Autodesk Fusion 360 part; units mm, degrees
sketch "Sketch1" plane through (0, 0, 0) normal (0, 0, 1) x (1, 0, 0)
  circle A0 centre (0, 0) radius 12.45
  dimension "d1" = 24.9
extrude "Extrude1" add sketch "Sketch1" along normal blind 18
sketch "Sketch2" plane through (0, 0, 18) normal (0, 0, 1) x (-1, 0, 0)
  circle A0 centre (0, 0) radius 12.45
  line L0 (0, 0) -> (0, -12.45)
  line L1 (0, 0) -> (-12.45, 0)
  line L2 (0, 0) -> (0, 12.45)
  line L3 (0, 0) -> (12.45, 0)
  line L4 (-12.45, 0) -> (-2.45, 0)
  circle A1 centre (-7.45, 0) radius 5
  line L5 (12.45, 0) -> (2.45, 0)
  line L6 (0, 12.45) -> (0, 2.45)
  line L7 (0, -12.45) -> (0, -2.45)
  circle A2 centre (0, -7.45) radius 5
  circle A3 centre (7.45, 0) radius 5
  circle A4 centre (0, 7.45) radius 5
  circle A5 centre (-7.45, 0) radius 3.75
  circle A6 centre (0, -7.45) radius 3.75
  circle A7 centre (0, 7.45) radius 3.75
  circle A8 centre (7.45, 0) radius 3.75
  circle A9 centre (-7.45, 0) radius 1
  circle A10 centre (0, -7.45) radius 1
  circle A11 centre (0, 7.45) radius 1
  circle A12 centre (7.45, 0) radius 1
  line L8 (-12.45, 0) -> (-12.45, -2.5)
  line L9 (-12.45, 0) -> (-12.45, 2.5)
  line L10 (-12.45, 2.5) -> (-11.7801, 2.5)
  line L11 (-12.45, -2.5) -> (-11.7801, -2.5)
  line L12 (0, -12.45) -> (-2.5, -12.45)
  line L13 (0, -12.45) -> (2.5, -12.45)
  line L14 (-2.5, -12.45) -> (-2.5, -11.7801)
  line L15 (12.45, 0) -> (12.45, -2.5)
  line L16 (12.45, 0) -> (12.45, 2.5)
  line L17 (12.45, 2.5) -> (10.2451, 2.5)
  line L18 (12.45, -2.5) -> (10.2451, -2.5)
  line L19 (2.5, -12.45) -> (2.5, -11.7801)
  line L20 (-2.5, -12.45) -> (-3.75, -12.45)
  line L21 (-3.75, -12.45) -> (-3.75, -10.7572)
  line L22 (2.5, -12.45) -> (3.75, -12.45)
  line L23 (3.75, -12.45) -> (3.75, -10.7572)
  line L24 (-3.75, -10.7572) -> (-3.75, -7.45)
  line L25 (2.5, -11.7801) -> (2.5, -10.2451)
  line L26 (-2.5, -11.7801) -> (-2.5, -10.2451)
  line L27 (3.75, -10.7572) -> (3.75, -7.45)
  line L28 (12.45, -2.5) -> (12.45, -3.75)
  line L29 (12.45, -3.75) -> (7.45, -3.75)
  line L30 (12.45, 1.25) -> (12.45, 2.5)
  line L31 (12.45, 2.5) -> (10.2451, 2.5)
  line L32 (12.45, 2.5) -> (12.45, 3.75)
  line L33 (12.45, 3.75) -> (7.45, 3.75)
  line L34 (0, 12.45) -> (-2.5, 12.45)
  line L35 (0, 12.45) -> (2.5, 12.45)
  line L36 (2.5, 12.45) -> (2.5, 10.2451)
  line L37 (2.5, 12.45) -> (3.75, 12.45)
  line L38 (3.75, 12.45) -> (3.75, 7.45)
  line L39 (-3.75, 7.45) -> (-3.75, 12.45)
  line L40 (-3.75, 12.45) -> (-2.5, 12.45)
  line L41 (-2.5, 12.45) -> (-2.5, 10.2451)
  line L42 (-11.7801, 2.5) -> (-10.2451, 2.5)
  line L43 (-11.7801, -2.5) -> (-10.2451, -2.5)
  line L44 (-12.45, -2.5) -> (-12.45, -3.75)
  line L45 (-12.45, 2.5) -> (-12.45, 3.75)
  line L46 (-12.45, 3.75) -> (-7.45, 3.75)
  line L47 (-12.45, -3.75) -> (-7.45, -3.75)
  dimension "d4" = 10
  dimension "d5" = 10
  dimension "d6" = 10
  dimension "d7" = 10
  dimension "d8" = 7.5
  dimension "d9" = 7.5
  dimension "d10" = 7.5
  dimension "d11" = 7.5
  dimension "d12" = 2
  dimension "d13" = 2
  dimension "d14" = 2
  dimension "d15" = 2
  dimension "d16" = 2.5
  dimension "d17" = 2.5
  dimension "d18" = 2.5
  dimension "d19" = 2.5
  dimension "d20" = 2.5
  dimension "d21" = 2.5
  dimension "d22" = 1.25
  dimension "d23" = 1.25
  dimension "d24" = 1.25
  dimension "d26" = 1.25
  dimension "d31" = 2.5
  dimension "d32" = 2.5
  dimension "d33" = 1.25
  dimension "d36" = 1.25
  dimension "d37" = 1.25
extrude "Extrude2" add sketch "Sketch2" along normal blind 14.44 contours A0 A2 L19 L23 | L0 L7 A2 A6 L27 | A2 A6 L25 L27 | L0 L7 A2 A6 L24 | A0 A2 L14 L21 | A2 A6 L24 L26 | L0 L7 A10 | L0 L7 A10
extrude "Extrude3" add sketch "Sketch2" along normal blind 14.44 contours A0 A3 L17 L31 L33 | A0 A3 L18 L29 | A3 A8 L17 L31 L33 | A3 A8 L18 L29 | L3 L5 A12 | L3 L5 A12 | L3 L5 A3 A8 L33 | L3 L5 A3 A8 L29
extrude "Extrude4" add sketch "Sketch2" along normal blind 14.44 contours A0 A4 L36 L38 | A4 A7 L36 L38 | L2 L6 A4 A7 L38 | L2 L6 A4 A7 L39 | A0 A4 L39 L41 | A4 A7 L39 L41 | L2 L6 A11 | L2 L6 A11
extrude "Extrude5" add sketch "Sketch2" along normal blind 14.44 contours L1 L4 A1 A5 L47 | L1 L4 A1 A5 L46 | A1 A5 L42 L46 | A0 A1 L10 L46 | A0 A1 L11 L47 | A1 A5 L43 L47 | L1 L4 A9 | L1 L4 A9
extrude "Extrude6" cut sketch "Sketch1" along normal blind 5
extrude "Extrude7" cut 1 faces at (3.0323, -6.4892, 5) along direction (0, 0, 1) blind 1.5
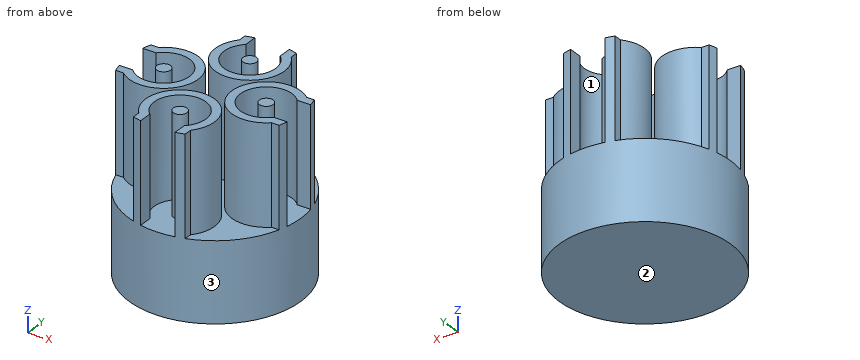
Geometry check sheet. Reference: the model listing, model coordinates, mm. Face numbers are marked on the shaded views. Round coordinates to 2 decimals unless told otherwise and drop trailing zeros. Loops run counter-clockwise (first coordinate to the right, second up) from the corner with the lowest first, then second, coordinate; pieces in that order, holes last.
Item 1: Cross-section at C-C on x = -7.45. Record the boundary of the cut face in (y, z).
Item 2: Cross-section at A-A on y = 0. Record the boundary of the cut face in (x, z), then the cut area to 3 significant figures.
Item 3: Thickness scan on line 1 (Y direction, x = 0, z = 25.75); line 2 (Y direction, x = 7.45, z = 25). Record the ranges inside material, lowest first.
Item 4: Gauge pin test, flat ends, axial feed: pin 1 (1.6 mm diameter, centred on y = 11.5, z = 23, fed in from +X); pin 2 (1.6 mm diameter, centred on x = -11, z = 25, fed in from +Y); pin 3 (1.5 mm diameter, centred on x = -8, y = 8.5, fed in from +Z); pin 4 (10 mm diameter, centred on y = 1.5, z = 9.5, fed in from -X). Record the tip position at first contact, or that the pin passes through.
Item 5: Mould release check, pull along X, two halves, no side actions. Record for the marked faces 1, 2 and 3: pulls with the +X half, pulls with the -X half, needs draft (parallel to the pull), parting line crosses it, or undercut.
Item 6: Cross-section at B-B on z = 30.25. Count the separate pieces of the cut face and the enclosed holes in it, then the cut area to 3 significant figures.
Answer sheet:
1. outline: (-9.97, 6.5) - (9.97, 6.5) - (9.97, 18) - (5, 18) - (5, 32.44) - (3.75, 32.44) - (3.75, 18) - (1, 18) - (1, 32.44) - (-1, 32.44) - (-1, 18) - (-3.75, 18) - (-3.75, 32.44) - (-5, 32.44) - (-5, 18) - (-9.97, 18) - close
2. outline: (-12.45, 6.5) - (12.45, 6.5) - (12.45, 18) - (8.45, 18) - (8.45, 32.44) - (6.45, 32.44) - (6.45, 18) - (3.7, 18) - (3.7, 32.44) - (2.45, 32.44) - (2.45, 18) - (-2.45, 18) - (-2.45, 32.44) - (-3.7, 32.44) - (-3.7, 18) - (-6.45, 18) - (-6.45, 32.44) - (-8.45, 32.44) - (-8.45, 18) - (-12.45, 18) - close
2. area: 380 mm2
3. line 1: y = -8.45 to -6.45, -3.7 to -2.45, 2.45 to 3.7, 6.45 to 8.45
3. line 2: y = -5 to -3.75, -1 to 1, 3.75 to 5
4. pin 1: stops at x = 3.8
4. pin 2: stops at y = 4.18
4. pin 3: stops at z = 18
4. pin 4: stops at x = -12.45
5. face 1: undercut
5. face 2: needs draft
5. face 3: parting line crosses it
6. separate pieces: 8
6. enclosed holes: 0
6. area: 131 mm2
